The model under review builds one solid part; all positions refer to its coordinate system, in mm. Face numbers are marked on the shaded views. A direction names the side the tool comes from. Round coordinates to 2 decimals unless told otherwise and drop trailing zeros. Write each loop counter-clockwise with the first axis right and the second up, starting at its lowest first coordinate (ties: lowest second). Pieces come first, ordered by that corner, then holes.
Item 1: Clearance check with flat-ended pins moving along their axes: pin 1 Ø8 at (x, z) = (30, -1) entering from +Y; pin 2 Ø2 at (x, z) = (44, -15) entering from +Y; pin 3 Ø2.5 at (x, z) = (40.5, 13.5) entering from -Y. State where each tip first meets the part, or that it passes through.
Item 2: Machinability: for the marked faces 1, 2 and 3, which of the approach directions +Z, -Z, +X, -X, +Y, -Y give a long, thin tool a straight path to every point of the face, cutting with its end or side? Answer none if there is none.
Item 3: Add section A-A (x = 36). Give the boundary of the cut face in (y, z), plus the area to 3 significant figures.
Item 4: Draft analysis for pull direction Z (two halves, no side actions). For the marked faces 4, 5 and 6, state which applies: +Z half, -Z half, draft (parallel to the pull), parting line (faces both ways), or undercut.
Item 5: To check wall thickness, follow L1, parallel to X at y = 4.5, z = 17; L2, parallel to Z at x = 25, y = 20; L3, parallel to Z at x = 34.5, y = 39. State the ranges of each line that lie inside material, in increasing order.
Item 6: Add section C-C (x = 29.5). Give the boundary of the cut face in (y, z), plus the area to 3 significant figures.
Item 7: Add section B-B (y = 4.5). State how many separate pieces and enclosed holes the cut face has, plus the area to 3 significant figures.
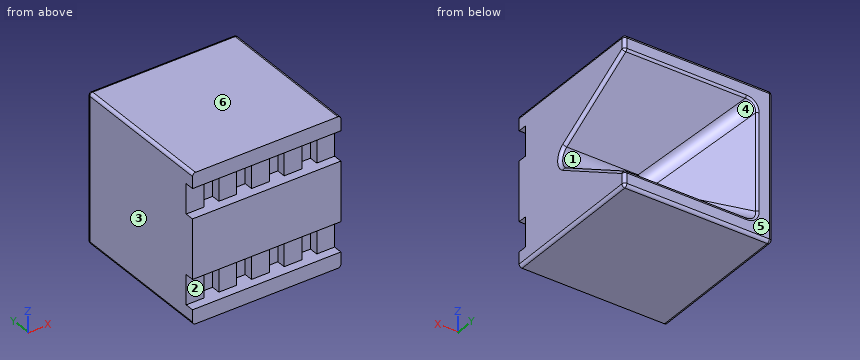
```python
from build123d import *

# Parameters (mm, degrees)
SKETCH1_W                = 50
SKETCH1_H                = 50
BOSS_EXTRUDE1_DEPTH      = 50
CUT_EXTRUDE1_DEPTH       = 50
BOSS_EXTRUDE2_DEPTH      = 25
BOSS_EXTRUDE2_DEPTH_BACK = 25
FILLET1_R                = 4
SKETCH4_W                = 50
SKETCH4_H                = 10
CUT_EXTRUDE3_DEPTH       = 3
SKETCH5_W                = 5
SKETCH5_H                = 10
CUT_EXTRUDE4_DEPTH       = 3
LPATTERN1_COUNT          = 4
LPATTERN1_PITCH          = 11
MIRROR1_COPY_1_SKETCH_W  = 5
MIRROR1_COPY_1_SKETCH_H  = 10
MIRROR1_COPY_1_DEPTH     = 3
MIRROR1_COPY_2_SKETCH_W  = 5
MIRROR1_COPY_2_SKETCH_H  = 10
MIRROR1_COPY_2_DEPTH     = 3
MIRROR1_COPY_3_SKETCH_W  = 5
MIRROR1_COPY_3_SKETCH_H  = 10
MIRROR1_COPY_3_DEPTH     = 3
FILLET2_R                = 1


with BuildPart() as part:
    # Sketch1 → Boss-Extrude1 (new body)
    with BuildSketch(Plane(origin=(0, 0, 0), x_dir=(1, 0, 0), z_dir=(0, 1, 0))):
        with Locations((25, 0)):
            Rectangle(SKETCH1_W, SKETCH1_H)
    extrude(amount=BOSS_EXTRUDE1_DEPTH)

    # Sketch2 → Cut-Extrude1 (cut)
    with BuildSketch(Plane(origin=(0, 0, 0), x_dir=(0, 0, -1), z_dir=(1, 0, 0))):
        Polygon((20, 50), (0, 15.358983849), (-20, 50), align=None)
    extrude(amount=CUT_EXTRUDE1_DEPTH, mode=Mode.SUBTRACT)

    # Sketch3 → Boss-Extrude2 (add, two sides)
    with BuildSketch(Plane.XY) as boss_extrude2_sk:
        Polygon((0, 50), (5, 50), (33.867513459, 0), (0, 0), align=None)
    extrude(amount=BOSS_EXTRUDE2_DEPTH)
    extrude(boss_extrude2_sk.sketch, amount=-BOSS_EXTRUDE2_DEPTH_BACK)

    # Fillet1
    fillet1_edges = [part.edges().sort_by_distance(p)[0] for p in [
        (37.5, 15.358983849, 0),
        (15, 32.679491924, -10),
        (15, 32.679491924, 10),
    ]]
    fillet(fillet1_edges, radius=FILLET1_R)

    # Sketch4 → Cut-Extrude3 (cut)
    with BuildSketch(Plane(origin=(0, 0, 0), x_dir=(1, 0, 0), z_dir=(0, 1, 0))):
        with Locations((25, -15)):
            Rectangle(SKETCH4_W, SKETCH4_H)
    cut_extrude3 = extrude(amount=CUT_EXTRUDE3_DEPTH, mode=Mode.SUBTRACT)

    # Sketch5 → Cut-Extrude4 (cut)
    with BuildSketch(Plane.XZ.offset(-3)):
        with Locations((8.5, 15)):
            Rectangle(SKETCH5_W, SKETCH5_H)
    cut_extrude4 = extrude(amount=-CUT_EXTRUDE4_DEPTH, mode=Mode.SUBTRACT)

    # LPattern1: Cut-Extrude4 ×4
    with Locations(*[(i * LPATTERN1_PITCH, 0, 0) for i in range(1, LPATTERN1_COUNT)]):
        add(cut_extrude4, mode=Mode.SUBTRACT)

    # Mirror1: Cut-Extrude4, Cut-Extrude3 across plane
    add(cut_extrude4.mirror(Plane.XY), mode=Mode.SUBTRACT)
    add(cut_extrude3.mirror(Plane.XY), mode=Mode.SUBTRACT)

    # Mirror1 copy 1 sketch → Mirror1 copy 1 (cut)
    with BuildSketch(Plane(origin=(11, 3, 0), x_dir=(1, 0, 0), z_dir=(0, -1, 0))):
        with Locations((8.5, -15)):
            Rectangle(MIRROR1_COPY_1_SKETCH_W, MIRROR1_COPY_1_SKETCH_H)
    extrude(amount=-MIRROR1_COPY_1_DEPTH, mode=Mode.SUBTRACT)

    # Mirror1 copy 2 sketch → Mirror1 copy 2 (cut)
    with BuildSketch(Plane(origin=(22, 3, 0), x_dir=(1, 0, 0), z_dir=(0, -1, 0))):
        with Locations((8.5, -15)):
            Rectangle(MIRROR1_COPY_2_SKETCH_W, MIRROR1_COPY_2_SKETCH_H)
    extrude(amount=-MIRROR1_COPY_2_DEPTH, mode=Mode.SUBTRACT)

    # Mirror1 copy 3 sketch → Mirror1 copy 3 (cut)
    with BuildSketch(Plane(origin=(33, 3, 0), x_dir=(1, 0, 0), z_dir=(0, -1, 0))):
        with Locations((8.5, -15)):
            Rectangle(MIRROR1_COPY_3_SKETCH_W, MIRROR1_COPY_3_SKETCH_H)
    extrude(amount=-MIRROR1_COPY_3_DEPTH, mode=Mode.SUBTRACT)

    # Fillet2
    fillet2_edges = [part.edges().sort_by_distance(p)[0] for p in [
        (50, 50, 22.5),
        (25, 50, -25),
        (50, 50, -22.5),
        (29.232050808, 50, -20),
        (29.232050808, 50, 20),
        (50, 35.679491924, 11.732050808),
        (0, 50, 0),
        (5, 50, 0),
        (50, 35.679491924, -11.732050808),
        (5.967318437, 50, -19.032681563),
        (5.967318437, 50, 19.032681563),
        (50, 19.358983849, 0),
        (25, 50, 25),
        (0, 25, -25),
        (50, 25, -25),
        (50, 25, 25),
        (0, 25, 25),
    ]]
    fillet(fillet2_edges, radius=FILLET2_R)


solid = part.part
```
Numbers:
1. pin 1: stops at y = 24.02
1. pin 2: stops at y = 43.07
1. pin 3: stops at y = 6
2. face 1: +X, +Y
2. face 2: +X, -X, -Y
2. face 3: +Z, -Z, -X, +Y, -Y
3. outline: (0, -25) - (49, -25) arc R1 ccw to (50, -24) - (50, -20.58) arc R1 ccw to (49.5, -19.71) - (21.36, -3.46) arc R4 cw to (21.36, 3.46) - (49.5, 19.71) arc R1 ccw to (50, 20.58) - (50, 24) arc R1 ccw to (49, 25) - (0, 25) - (0, 20) - (3, 20) - (3, 10) - (0, 10) - (0, -10) - (3, -10) - (3, -20) - (0, -20) - close
3. area: 1,760 mm2
4. face 4: undercut
4. face 5: draft
4. face 6: +Z half
5. L1: x = 0 to 6, 11 to 17, 22 to 28, 33 to 39, 44 to 50
5. L2: z = -25 to -2.17, 2.17 to 25
5. L3: z = -25 to -13.65, 13.65 to 25
6. outline: (0, -25) - (49, -25) arc R1 ccw to (50, -24) - (50, -20.58) arc R1 ccw to (49.5, -19.71) - (21.36, -3.46) arc R4 cw to (21.36, 3.46) - (49.5, 19.71) arc R1 ccw to (50, 20.58) - (50, 24) arc R1 ccw to (49, 25) - (0, 25) - (0, 20) - (6, 20) - (6, 10) - (0, 10) - (0, -10) - (6, -10) - (6, -20) - (0, -20) - close
6. area: 1,700 mm2
7. separate pieces: 1
7. enclosed holes: 8
7. area: 2,100 mm2
